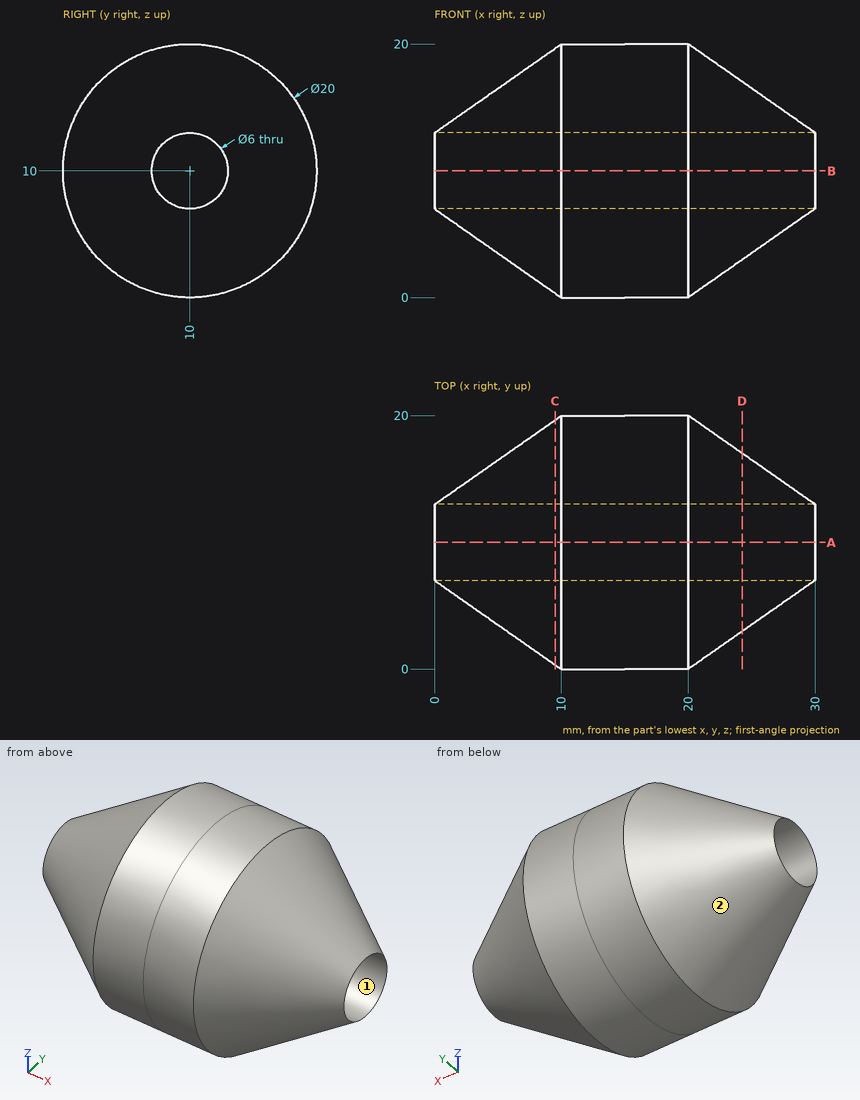
Could you check a few things on this drawing? It's one solid part, dimensions in mm from its lowest x, y, z. Round coordinates to 2 decimals unless told otherwise and drop trailing zeros. Write each loop counter-clockwise with the first axis right and the second up, starting at its lowest first coordinate (ties: lowest second). Pieces come first, ordered by that corner, then holes. Notation, with made-up numbers: (85, 25.5) -> (131, 25.5) arc R17 ccw to (131, 31.5) -> close; hole circle Ø5 at (39, 75). An arc over 180 degrees is marked (long way). One line per item, written item: value.
1) Suppose I cut it at C-C on x = 9.5. List the corners of the cut face in (y, z) for me.
Filled sheet:
outline: circle Ø19.3 at (10, 10); hole circle Ø6 at (10, 10)
2) I'm going to push flat-ended pins straight in: pin 1 Ø5 at (y, z) = (2.5, 12.5) entering from +X; pin 2 Ø1.5 at (x, z) = (9, 13.5) entering from -Y; pin 3 Ø1 at (x, y) = (10, 8) entering from -Z. Where does each tip first touch, or does it pass through?
Filled sheet:
pin 1: stops at x = 26.56
pin 2: stops at y = 0.76
pin 3: stops at z = 0.11
3) Suppose I cut it at D-D on x = 24.25. List the corners of the cut face in (y, z) for me (3 decimals), plus the area to 3 significant figures.
Filled sheet:
outline: circle Ø14.05 at (10, 10); hole circle Ø6 at (10, 10)
area: 127 mm2
4) If I drill on line 1 (Z direction, x = 21.5, y = 10); line 2 (Y direction, x = 20.75, z = 10) (3 decimals); line 3 (Z direction, x = 18.5, y = 12), over which ranges is the centre line in solid material (lowest first)? Write a range as [from, to].
Filled sheet:
line 1: z = [1.05, 7], [13, 18.95]
line 2: y = [0.525, 7], [13, 19.475]
line 3: z = [0.2, 7.76], [12.24, 19.8]
5) Suppose I cut it at A-A on y = 10. List the corners of the cut face in (x, z) for me, plus the area to 3 significant figures.
Filled sheet:
outline: (0, 7) -> (10, 0) -> (20, 0) -> (30, 7) -> close; (0, 13) -> (30, 13) -> (20, 20) -> (10, 20) -> close
area: 280 mm2
6) We'd pull the mould along Y, two halves only. Please class the marked faces 1 and 2: released by +Y, released by -Y, zero draft, split by the parting line, or undercut.
Filled sheet:
face 1: undercut
face 2: split by the parting line
